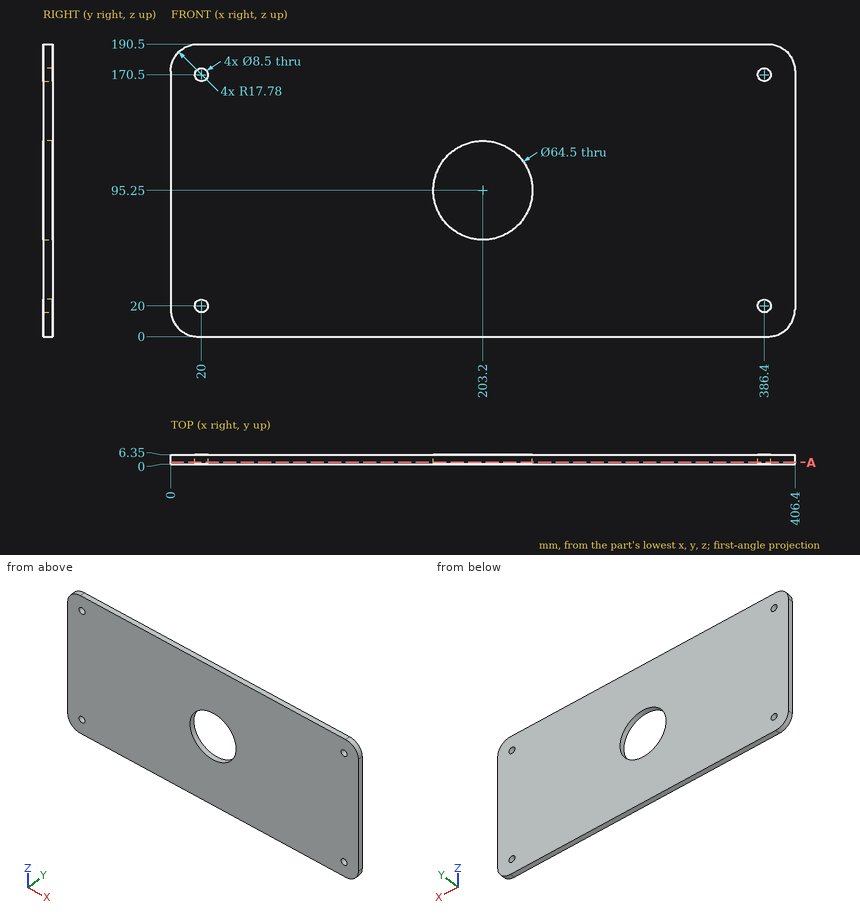
Here's the drawing with two shaded views (mm, measured from the low corner). I have some questions. Give positions to 0.01 mm unless a question says otherwise; leave off trailing zeros. Order: outer loops, then holes, each group sorted by start corner. A loop starts at its lowest first (then second) coordinate and runs counter-clockwise, first axis right, second up. Notation, with made-up numbers: (89.5, 16) - (110.5, 16) arc R17 ccw to (110.5, 30) - close; hole circle Ø4 at (4, 34). An arc over 180 degrees is marked (long way). Use a Markdown table: item, result. Add a question column.
Q1. If we section it at A-A on y = 1.25: Write out the boundary of the cut face in (x, z), plus the area to 3 significant figures.
Q2. Please list where these lines run through material, in increasing order: line 1 along X through (y, z) = (5.25, 20); line 2 along Z through (x, y) = (386.4, 3); line 3 along X through (y, z) = (3.5, 95.25).
Q3. I'm going to push a flat-ended pin straight in: pin 1 (7 mm diameter, centred on x = 386.4, z = 170.5, fed in from -Y). Where does the tip first touch, or does it pass through?
Answers follow:
| question | item | result |
|---|---|---|
| 1 | outline | (0, 17.78) arc R17.78 ccw to (17.78, 0) - (388.62, 0) arc R17.78 ccw to (406.4, 17.78) - (406.4, 172.72) arc R17.78 ccw to (388.62, 190.5) - (17.78, 190.5) arc R17.78 ccw to (0, 172.72) - close; hole circle Ø8.5 at (20, 20); hole circle Ø8.5 at (20, 170.5); hole circle Ø64.5 at (203.2, 95.25); hole circle Ø8.5 at (386.4, 20); hole circle Ø8.5 at (386.4, 170.5) |
| 1 | area | 73,700 mm^2 |
| 2 | line 1 | x = 0 to 15.75, 24.25 to 382.15, 390.65 to 406.4 |
| 2 | line 2 | z = 0 to 15.75, 24.25 to 166.25, 174.75 to 190.5 |
| 2 | line 3 | x = 0 to 170.95, 235.45 to 406.4 |
| 3 | pin 1 | passes through |
